```python
from build123d import *

# Parameters (mm, degrees)
F1_DEPTH     = 30
F2_R         = 10
F3_W         = 20
F3_H         = 1
F4_DEPTH     = 4
F6_DEPTH     = 3
F7_T1_DEPTH  = 26.6017443282
F8_T1_DEPTH  = 30.2743860668
F9_W         = 2
F9_H         = 3
F11_DEPTH    = 2
F10_W        = 2
F10_H        = 3
F12_DEPTH    = 2
F13_SIZE     = 1.99999
F14_T1_DEPTH = 10.6602829052
F14_T3_DEPTH = 10.6602829052


# Not quite as in the source:
# - a fillet or chamfer that OpenCascade refuses, or shapes differently, is made with other operations: its cross-section is extruded or revolved along the edge and cut away or added
# - a fillet or chamfer is up to 0.001 mm smaller than in the source, because OpenCascade refuses the exact size


with BuildPart() as f1:
    # F0 (on Right) → F1 (new body, symmetric)
    with BuildSketch(Plane.YZ):
        with BuildLine():
            Line((-2, 0), (0, 0))
            Line((0, 0), (0, 28.5))
            ThreePointArc((0, 28.5), (-3.3682720164, 36.6317279836), (-11.5, 40))
            Line((-11.5, 40), (-26.5, 40))
            ThreePointArc((-26.5, 40), (-34.6317279836, 36.6317279836), (-38, 28.5))
            Line((-38, 28.5), (-38, 0))
            Line((-38, 0), (-36, 0))
            Line((-36, 0), (-36, 28.5))
            ThreePointArc((-36, 28.5), (-32.9045321983, 35.2456883731), (-26.0125078223, 38))
            Line((-26.0125078223, 38), (-11.9874921777, 38))
            ThreePointArc((-11.9874921777, 38), (-5.0954678017, 35.2456883731), (-2, 28.5))
            Line((-2, 28.5), (-2, 0))
        make_face()
    extrude(amount=F1_DEPTH, both=True)

    # F2
    f2_edges = [f1.edges().sort_by_distance(p)[0] for p in [
        (30, -37, 0),
        (30, -1, 0),
        (-30, -1, 0),
        (-30, -37, 0),
    ]]
    fillet(f2_edges, radius=F2_R)

    # F3 (on face) → F4 (join)
    with BuildSketch(Plane(origin=(0, 0, 0), x_dir=(1, 0, 0), z_dir=(0, 0, -1))):
        with Locations((0, 0.5)):
            Rectangle(F3_W, F3_H)
        with Locations((0, 37.5)):
            Rectangle(F3_W, F3_H)
    extrude(amount=F4_DEPTH)

    # F5 (on face) → F6 (join)
    with BuildSketch(Plane(origin=(0, 0, -4), x_dir=(1, 0, 0), z_dir=(0, 0, -1))):
        Polygon((10, 38), (-10, 38), (-10, 36.5000508078), (9.987654115, 36.5000508078), align=None)
        Polygon((-10, 1.4999491922), (-10, 0), (10, 0), (9.987654115, 1.4999491922), align=None)
    extrude(amount=F6_DEPTH)

    # F7: fillet of radius 2 on 2 edges, made by hand

    # F7_s2 → F7_t1 (cut)
    with BuildSketch(Plane.YZ.offset(-13.3070451066)):
        with BuildLine():
            ThreePointArc((-1.4999491922, -5.3228180426), (-1.3707914645, -4.6157471889), (-1, -4))
            Line((-1, -4), (-1.4999491922, -4))
            Line((-1.4999491922, -4), (-1.4999491922, -5.3228180426))
        make_face()
        with BuildLine():
            ThreePointArc((-37, -4), (-36.6292085355, -4.6157471889), (-36.5000508078, -5.3228180426))
            Line((-36.5000508078, -5.3228180426), (-36.5000508078, -4))
            Line((-36.5000508078, -4), (-37, -4))
        make_face()
    extrude(amount=F7_T1_DEPTH, mode=Mode.SUBTRACT)

    # F8: chamfer of 2 on 2 edges, made by hand

    # F8_s2 → F8_t1 (cut)
    with BuildSketch(Plane.YZ.offset(-15.1433659759)):
        Polygon((0.5000508078, -7), (-1.4999491922, -5), (-1.4999491922, -7), align=None)
        Polygon((-38.5000508078, -7), (-36.5000508078, -5), (-36.5000508078, -7), align=None)
    extrude(amount=F8_T1_DEPTH, mode=Mode.SUBTRACT)

    # F9 (on face) → F11 (join)
    with BuildSketch(Plane.XZ.offset(2)):
        Polygon((-25, 11), (-25, 10), (-25, 9), (-22, 9), (-22, 11), align=None)
        with Locations((-23.5, 14.5)):
            Rectangle(F9_W, F9_H)
        Polygon((-5, 9), (-5, 10), (-5, 11), (-8, 11), (-8, 9), align=None)
        with Locations((-6.5, 14.5)):
            Rectangle(F9_W, F9_H)
    extrude(amount=F11_DEPTH)

    # F10 (on face) → F12 (join)
    with BuildSketch(Plane(origin=(0, -36, 0), x_dir=(-1, 0, 0), z_dir=(0, 1, 0))):
        Polygon((22, 11), (22, 10), (22, 9), (25, 9), (25, 11), align=None)
        with Locations((23.5, 14.5)):
            Rectangle(F10_W, F10_H)
        Polygon((8, 9), (8, 10), (8, 11), (5, 11), (5, 9), align=None)
        with Locations((6.5, 14.5)):
            Rectangle(F10_W, F10_H)
    extrude(amount=F12_DEPTH)

    # F13 (size 2 in the source; OpenCascade refuses exactly that, so slightly less here)
    f13_edges = [f1.edges().sort_by_distance(p)[0] for p in [
        (-23.5, -4, 16),
        (-23.5, -34, 16),
        (-6.5, -4, 16),
        (-6.5, -34, 16),
    ]]
    chamfer(f13_edges, length=F13_SIZE)

    # F14: fillet of radius 2 on 4 edges, made by hand

    # F14_s2 → F14_t1 (cut)
    with BuildSketch(Plane.YZ.offset(-28.8301414526)):
        with BuildLine():
            ThreePointArc((-4, 14.00001), (-3.267948419, 13.2679520792), (-2.267943419, 13))
            Line((-2.267943419, 13), (-4, 13))
            Line((-4, 13), (-4, 14.00001))
        make_face()
        with BuildLine():
            ThreePointArc((-35.732056581, 13), (-34.732051581, 13.2679520792), (-34, 14.00001))
            Line((-34, 14.00001), (-34, 13))
            Line((-34, 13), (-35.732056581, 13))
        make_face()
    extrude(amount=F14_T1_DEPTH, mode=Mode.SUBTRACT)

    # F14_s4 → F14_t3 (cut)
    with BuildSketch(Plane.YZ.offset(-11.8301414526)):
        with BuildLine():
            ThreePointArc((-2.267943419, 13), (-3.267948419, 13.2679520792), (-4, 14.00001))
            Line((-4, 14.00001), (-4, 13))
            Line((-4, 13), (-2.267943419, 13))
        make_face()
        with BuildLine():
            ThreePointArc((-35.732056581, 13), (-34.732051581, 13.2679520792), (-34, 14.00001))
            Line((-34, 14.00001), (-34, 13))
            Line((-34, 13), (-35.732056581, 13))
        make_face()
    extrude(amount=F14_T3_DEPTH, mode=Mode.SUBTRACT)


solid = f1.part
```
Part model, mm, in its own coordinate system. A direction names the side the tool comes from. Round coordinates to 2 decimals unless told otherwise and drop trailing zeros. Loops run counter-clockwise (first coordinate to the right, second up) from the corner with the lowest first, then second, coordinate; pieces in that order, holes last. Notation, with made-up numbers: (-26, -9) -> (14, -9) arc R17 cw to (14, 9) -> close; hole circle Ø3 at (53, -5). An arc over 180 degrees is marked (long way). Use one line per item in the form item = value. Start each with the question number.
Item 1: Band-saw the part on A-A (z = 23.5). List the corners of the cut face in (x, y), plus the area to 3 significant figures.
Item 2: Tool access for faces 5 (the flat face through (-23, -34, 10)), 6 (the flat face through (0.3, -36.8, 0)), 7 (the cylindrical face through (-23.514, -34.745, 13.261)): list every direction of +Z, -Z, +X, -X, +Y, -Y with a clear straight run to the whole face (end or side of a thin tool).
Item 3: Drop flat-ended pins along their axis: pin 1 Ø5 at (x, z) = (-2.5, 32) entering from -Y; pin 2 Ø3 at (x, y) = (0, -23.5) entering from -Z; pin 3 Ø3 at (x, y) = (-21.5, -6) entering from +Z. Give the stop position or say it passes through.
Item 4: Band-saw the part on C-C (z = 30.5). List the corners of the cut face in (x, y), plus the area to 3 significant figures.
Item 5: Band-saw the part on B-B (x = -13). List the corners of the cut face in (y, z), plus the area to 3 significant figures.
Item 6: Drill centre lines: line 1 along Y through (x, z) = (5, 16.5); line 2 along Y through (x, z) = (-21, 33); line 3 along Z through (x, y) = (8, -26.5). Where is each one in solid material? Low to high.
Item 7: Band-saw the part on D-D (y = -13). List the corners of the cut face in (x, z), plus the area to 3 significant figures.
Item 8: Two-plate mould, pull along X, no slides. Class faces 1 (the flat face through (-22, -3, 10)), 2 (the flat face through (-8, -35, 10)), 3 (the flat face through (-24.5, -35, 14)), 4 (the flat face through (-0.1, -0.7, -5.8)): released by +X, released by -X, zero draft, split by the parting line, or undercut.
Data:
q1.outline = (-30, -38) -> (30, -38) -> (30, -36) -> (-30, -36) -> close; (-30, -2) -> (30, -2) -> (30, 0) -> (-30, 0) -> close
q1.area = 240 mm^2
q2.face_5 = -Z, +X, -X
q2.face_6 = none
q2.face_7 = +X, -X
q3.pin_1 = -37.96
q3.pin_2 = 38
q3.pin_3 = 39.28
q4.outline = (-30, -37.82) -> (30, -37.82) -> (30, -35.69) -> (-30, -35.69) -> close; (-30, -2.31) -> (30, -2.31) -> (30, -0.18) -> (-30, -0.18) -> close
q4.area = 256 mm^2
q5.outline = (-38, 0) -> (-36, 0) -> (-36, 28.5) arc R10 cw to (-26.01, 38) -> (-11.99, 38) arc R10 cw to (-2, 28.5) -> (-2, 0) -> (0, 0) -> (0, 28.5) arc R11.5 ccw to (-11.5, 40) -> (-26.5, 40) arc R11.5 ccw to (-38, 28.5) -> close
q5.area = 214 mm^2
q6.line_1 = -38 to -36, -2 to 0
q6.line_2 = -37.08 to -34.67, -3.33 to -0.92
q6.line_3 = 37.99 to 40
q7.outline = (-30, 38) -> (30, 38) -> (30, 40) -> (-30, 40) -> close
q7.area = 120 mm^2
q8.face_1 = undercut
q8.face_2 = undercut
q8.face_3 = released by -X
q8.face_4 = zero draft
